Geometry: final body of the model. Coordinates: model frame, mm. Round coordinates to 2 decimals unless told otherwise and drop trailing zeros. Order: outer loops, then holes, each group sorted by start corner. A loop starts at its lowest first (then second) coordinate and runs counter-clockwise, first axis right, second up. Notation, with made-up numbers: (53.25, 64) - (108.25, 64) arc R17 cw to (108.25, 85) - close; hole circle Ø7 at (-40, 73). An arc over 180 degrees is marked (long way). Put each result on its own line as item: value. Start each with the question number.
(1) Pin query (flat end, axial travel): P1, Ø4.5, axis at y = 0, z = -20, coming from the -X side; P2, Ø1, axis at x = 0.5, y = -13, coming from the -Z side. Return the tip coordinate at first contact, or that it passes through.
(2) Section B-B (y = 0). Output: boundary loops of the cut face in (x, z), and give its area (3 significant figures).
(3) Material intervals for L1, parallel to Y at x = 2.5, z = -20; L2, parallel to Z at x = 2.75, y = 0; L3, parallel to Z at x = 2.15, y = 1, sorted ascending. Write a range as [from, to].
(4) Pull-direction query (Y, two-part tool) for faces 1 (the face through (0.872, 19.227, -39.145)), 2 (the face through (1.92, 0.64, -17.97)), 3 (the face through (3, 1.2, -21.6)), 4 (the face through (0.62, 0.26, -39.37)); classes: released by +Y, released by -Y, zero draft, split by the parting line, or undercut.
(5) Section A-A (z = -20). Output: boundary loops of the cut face in (x, y).
Autodesk Inventor part; units mm, degrees
ref_plane "CS_ANBAU_CAP_XY" through (0, 0, 0) normal (0, 1, 0) x (1, 0, 0)
ref_plane "CS_ANBAU_CAP_YZ" through (0, 0, 0) normal (1, 0, 0) x (0, 0, -1)
ref_plane "CS_ANBAU_CAP_ZX" through (0, 0, 0) normal (0, 0, -1) x (0, 1, 0)
sketch "Skizze_1" plane through (0, 0, 0) normal (1, 0, 0) x (0, 0, -1)
  line L0 (-40, 20) -> (-40, -20)
  line L1 (-40, -20) -> (40, -20)
  line L2 (40, -20) -> (40, 20)
  line L3 (40, 20) -> (-40, 20)
extrude "Extrusion1" add sketch "Skizze_1" along normal blind 4
sketch "Sketch2" plane through (0, 0, 0) normal (-1, 0, 0) x (0, 0, 1)
  point P0 (20, 0)
hole "Hole1" at (0, 0, 20) direction (1, 0, 0) diameter 4 depth 4 countersink diameter 8.1 countersink angle 90
sketch "Sketch3" plane through (0, 0, 0) normal (-1, 0, 0) x (0, 0, 1)
  point P0 (-20, 0)
hole "Hole2" at (0, 0, -20) direction (1, 0, 0) diameter 4 depth 4 countersink diameter 8.1 countersink angle 90
ref_plane "CS_ANBAU_CAP_XY" through (0, 0, 0) normal (0, 1, 0) x (1, 0, 0)
ref_plane "CS_ANBAU_CAP_YZ" through (0, 0, 0) normal (1, 0, 0) x (0, 0, -1)
ref_plane "CS_ANBAU_CAP_ZX" through (0, 0, 0) normal (0, 0, -1) x (0, 1, 0)
ref_plane "CS_ANBAU_CAP_90_XY" through (0, 0, 0) normal (0, 0, 1) x (1, 0, 0)
ref_plane "CS_ANBAU_CAP_90_YZ" through (0, 0, 0) normal (1, 0, 0) x (0, 1, 0)
ref_plane "CS_ANBAU_CAP_90_ZX" through (0, 0, 0) normal (0, 1, 0) x (0, 0, 1)
ref_plane "IB_1_XY" through (0, 0, 0) normal (1, 0, 0) x (0, 0, -1)
ref_plane "IB_1_YZ" through (0, 0, 0) normal (0, 0, -1) x (0, 1, 0)
ref_plane "IB_1_ZX" through (0, 0, 0) normal (0, 1, 0) x (1, 0, 0)
ref_plane "IB_10_XY" through (0, -14, 30) normal (1, 0, 0) x (0, 0, -1)
ref_plane "IB_10_YZ" through (0, -14, 30) normal (0, 0, -1) x (0, 1, 0)
ref_plane "IB_10_ZX" through (0, -14, 30) normal (0, 1, 0) x (1, 0, 0)
ref_plane "IB_11_XY" through (0, 14, 30) normal (1, 0, 0) x (0, 0, -1)
ref_plane "IB_11_YZ" through (0, 14, 30) normal (0, 0, -1) x (0, 1, 0)
ref_plane "IB_11_ZX" through (0, 14, 30) normal (0, 1, 0) x (1, 0, 0)
ref_plane "IB_12_XY" through (0, 0, -20) normal (1, 0, 0) x (0, 0, -1)
ref_plane "IB_12_YZ" through (0, 0, -20) normal (0, 0, -1) x (0, 1, 0)
ref_plane "IB_12_ZX" through (0, 0, -20) normal (0, 1, 0) x (1, 0, 0)
ref_plane "IB_2_XY" through (0, 0, -20) normal (1, 0, 0) x (0, 0, -1)
ref_plane "IB_2_YZ" through (0, 0, -20) normal (0, 0, -1) x (0, 1, 0)
ref_plane "IB_2_ZX" through (0, 0, -20) normal (0, 1, 0) x (1, 0, 0)
ref_plane "IB_3_XY" through (0, 0, 20) normal (1, 0, 0) x (0, 0, -1)
ref_plane "IB_3_YZ" through (0, 0, 20) normal (0, 0, -1) x (0, 1, 0)
ref_plane "IB_3_ZX" through (0, 0, 20) normal (0, 1, 0) x (1, 0, 0)
ref_plane "IB_4_XY" through (0, 13.5, -33.5) normal (1, 0, 0) x (0, 0, -1)
ref_plane "IB_4_YZ" through (0, 13.5, -33.5) normal (0, 0, -1) x (0, 1, 0)
ref_plane "IB_4_ZX" through (0, 13.5, -33.5) normal (0, 1, 0) x (1, 0, 0)
ref_plane "IB_5_XY" through (0, 13.5, 33.5) normal (1, 0, 0) x (0, 0, -1)
ref_plane "IB_5_YZ" through (0, 13.5, 33.5) normal (0, 0, -1) x (0, 1, 0)
ref_plane "IB_5_ZX" through (0, 13.5, 33.5) normal (0, 1, 0) x (1, 0, 0)
ref_plane "IB_6_XY" through (0, 1.5, 26.5) normal (1, 0, 0) x (0, 0, -1)
ref_plane "IB_6_YZ" through (0, 1.5, 26.5) normal (0, 0, -1) x (0, 1, 0)
ref_plane "IB_6_ZX" through (0, 1.5, 26.5) normal (0, 1, 0) x (1, 0, 0)
ref_plane "IB_7_XY" through (0, 1.5, -26.5) normal (1, 0, 0) x (0, 0, -1)
ref_plane "IB_7_YZ" through (0, 1.5, -26.5) normal (0, 0, -1) x (0, 1, 0)
ref_plane "IB_7_ZX" through (0, 1.5, -26.5) normal (0, 1, 0) x (1, 0, 0)
ref_plane "IB_8_XY" through (0, -2, 34) normal (1, 0, 0) x (0, 0, -1)
ref_plane "IB_8_YZ" through (0, -2, 34) normal (0, 0, -1) x (0, 1, 0)
ref_plane "IB_8_ZX" through (0, -2, 34) normal (0, 1, 0) x (1, 0, 0)
ref_plane "IB_9_XY" through (0, -2, -34) normal (1, 0, 0) x (0, 0, -1)
ref_plane "IB_9_YZ" through (0, -2, -34) normal (0, 0, -1) x (0, 1, 0)
ref_plane "IB_9_ZX" through (0, -2, -34) normal (0, 1, 0) x (1, 0, 0)
chamfer "Chamfer1" distance 1.25 angle 45 8 edges at (2, -20, 40) (0, -20, 0) (0, 0, 40) (2, -20, -40) (0, 0, -40) (2, 20, -40) (0, 20, 0) (2, 20, 40)
sketch "Sketch5" plane through (4, 0, 0) normal (1, 0, 0) x (0, 0, -1)
  line L0 (-38.75, -20) -> (38.75, -20)
  line L1 (-12, -20) -> (-40, -20)
  line L2 (-40, -20) -> (-40, 20)
  line L3 (-40, 20) -> (-12, 20)
  line L4 (-12, 20) -> (-12, -20)
  line L5 (-40, 18.75) -> (-40, -18.75)
  line L6 (38.75, 20) -> (-38.75, 20)
  line L7 (40, -18.75) -> (40, 18.75)
  point P0 (0, 0)
  dimension "d32" = 52
extrude "Extrusion2" cut sketch "Sketch5" against normal through all
properties part number "Robotunits CAP_4080_1" material "ABS PlastiK"
Checks:
1. P1: stops at x = 1.8
1. P2: stops at z = -39.75
2. outline: (0, -38.75) - (1.25, -40) - (4, -40) - (4, -22) - (2.05, -22) - (0, -24.05) - close; (0, -15.95) - (2.05, -18) - (4, -18) - (4, 12) - (0, 12) - close
2. area: 187 mm²
3. L1: y = [-20, -2], [2, 20]
3. L2: z = [-40, -22], [-18, 12]
3. L3: z = [-40, -21.73], [-18.27, 12]
4. face 1: released by +Y
4. face 2: undercut
4. face 3: undercut
4. face 4: zero draft
5. outline: (0, -18.75) - (1.25, -20) - (4, -20) - (4, -2) - (2.05, -2) - (0, -4.05) - close; (0, 4.05) - (2.05, 2) - (4, 2) - (4, 20) - (1.25, 20) - (0, 18.75) - close
